```python
from build123d import *

# Parameters (mm, degrees)
SKETCH1_R                   = 250
SKETCH1_R_2                 = 25
BOSS_EXTRUDE1_DEPTH         = 6.35
TAP_DRILL_FOR_M4X0_7_TAP1_D = 3.3
TAP_DRILL_FOR_M6X1_0_TAP1_D = 5


with BuildPart() as part:
    # Sketch1 → Boss-Extrude1 (new body)
    with BuildSketch(Plane(origin=(0, 0, 0), x_dir=(1, 0, 0), z_dir=(0, 1, 0))):
        with Locations(Location((0, 0, 0), (0, 0, 270))):
            Circle(SKETCH1_R)
        with Locations(Location((0, 0, 0), (0, 0, 270))):
            Circle(SKETCH1_R_2, mode=Mode.SUBTRACT)
        with BuildLine():
            Line((-51.699063768, 192.943532686), (-21.846841855, 81.533523786))
            ThreePointArc((-21.846841855, 81.533523786), (-22.566264891, 74.464334994), (-27.799500104, 69.65764706))
            ThreePointArc((-27.799500104, 69.65764706), (-37.5, 64.951905284), (-46.42554187, 58.903896832))
            ThreePointArc((-46.42554187, 58.903896832), (-53.204873335, 56.775126162), (-59.686681932, 59.686681932))
            Line((-59.686681932, 59.686681932), (-141.244468918, 141.244468918))
            ThreePointArc((-141.244468918, 141.244468918), (-144.170273662, 148.565614941), (-140.882071162, 155.731313567))
            ThreePointArc((-140.882071162, 155.731313567), (-105, 181.865334795), (-64.426238133, 199.873109347))
            ThreePointArc((-64.426238133, 199.873109347), (-56.576459837, 199.137926932), (-51.699063768, 192.943532686))
        make_face(mode=Mode.SUBTRACT)
        with BuildLine():
            Line((141.244468918, 141.244468918), (59.686681932, 59.686681932))
            ThreePointArc((59.686681932, 59.686681932), (53.204873335, 56.775126162), (46.42554187, 58.903896832))
            ThreePointArc((46.42554187, 58.903896832), (37.5, 64.951905284), (27.799500104, 69.65764706))
            ThreePointArc((27.799500104, 69.65764706), (22.566264891, 74.464334994), (21.846841855, 81.533523786))
            Line((21.846841855, 81.533523786), (51.699063768, 192.943532686))
            ThreePointArc((51.699063768, 192.943532686), (56.576459837, 199.137926932), (64.426238133, 199.873109347))
            ThreePointArc((64.426238133, 199.873109347), (105, 181.865334795), (140.882071162, 155.731313567))
            ThreePointArc((140.882071162, 155.731313567), (144.170273662, 148.565614941), (141.244468918, 141.244468918))
        make_face(mode=Mode.SUBTRACT)
        with BuildLine():
            Line((192.943532686, -51.699063768), (81.533523786, -21.846841855))
            ThreePointArc((81.533523786, -21.846841855), (75.771138227, -17.689208833), (74.225041974, -10.753750228))
            ThreePointArc((74.225041974, -10.753750228), (75, 0), (74.225041974, 10.753750228))
            ThreePointArc((74.225041974, 10.753750228), (75.771138227, 17.689208833), (81.533523786, 21.846841855))
            Line((81.533523786, 21.846841855), (192.943532686, 51.699063768))
            ThreePointArc((192.943532686, 51.699063768), (200.746733498, 50.572311991), (205.308309294, 44.14179578))
            ThreePointArc((205.308309294, 44.14179578), (210, 0), (205.308309294, -44.14179578))
            ThreePointArc((205.308309294, -44.14179578), (200.746733498, -50.572311991), (192.943532686, -51.699063768))
        make_face(mode=Mode.SUBTRACT)
        with BuildLine():
            Line((51.699063768, -192.943532686), (21.846841855, -81.533523786))
            ThreePointArc((21.846841855, -81.533523786), (22.566264891, -74.464334994), (27.799500104, -69.65764706))
            ThreePointArc((27.799500104, -69.65764706), (37.5, -64.951905284), (46.42554187, -58.903896832))
            ThreePointArc((46.42554187, -58.903896832), (53.204873335, -56.775126162), (59.686681932, -59.686681932))
            Line((59.686681932, -59.686681932), (141.244468918, -141.244468918))
            ThreePointArc((141.244468918, -141.244468918), (144.170273662, -148.565614941), (140.882071162, -155.731313567))
            ThreePointArc((140.882071162, -155.731313567), (105, -181.865334795), (64.426238133, -199.873109347))
            ThreePointArc((64.426238133, -199.873109347), (56.576459837, -199.137926932), (51.699063768, -192.943532686))
        make_face(mode=Mode.SUBTRACT)
        with BuildLine():
            Line((-141.244468918, -141.244468918), (-59.686681932, -59.686681932))
            ThreePointArc((-59.686681932, -59.686681932), (-53.204873335, -56.775126162), (-46.42554187, -58.903896832))
            ThreePointArc((-46.42554187, -58.903896832), (-37.5, -64.951905284), (-27.799500104, -69.65764706))
            ThreePointArc((-27.799500104, -69.65764706), (-22.566264891, -74.464334994), (-21.846841855, -81.533523786))
            Line((-21.846841855, -81.533523786), (-51.699063768, -192.943532686))
            ThreePointArc((-51.699063768, -192.943532686), (-56.576459837, -199.137926932), (-64.426238133, -199.873109347))
            ThreePointArc((-64.426238133, -199.873109347), (-105, -181.865334795), (-140.882071162, -155.731313567))
            ThreePointArc((-140.882071162, -155.731313567), (-144.170273662, -148.565614941), (-141.244468918, -141.244468918))
        make_face(mode=Mode.SUBTRACT)
        with BuildLine():
            Line((-192.943532686, 51.699063768), (-81.533523786, 21.846841855))
            ThreePointArc((-81.533523786, 21.846841855), (-75.771138227, 17.689208833), (-74.225041974, 10.753750228))
            ThreePointArc((-74.225041974, 10.753750228), (-75, 0), (-74.225041974, -10.753750228))
            ThreePointArc((-74.225041974, -10.753750228), (-75.771138227, -17.689208833), (-81.533523786, -21.846841855))
            Line((-81.533523786, -21.846841855), (-192.943532686, -51.699063768))
            ThreePointArc((-192.943532686, -51.699063768), (-200.746733498, -50.572311991), (-205.308309294, -44.14179578))
            ThreePointArc((-205.308309294, -44.14179578), (-210, 0), (-205.308309294, 44.14179578))
            ThreePointArc((-205.308309294, 44.14179578), (-200.746733498, 50.572311991), (-192.943532686, 51.699063768))
        make_face(mode=Mode.SUBTRACT)
    extrude(amount=-BOSS_EXTRUDE1_DEPTH)

    # Tap Drill for M4x0.7 Tap1 (through all)
    with Locations(Plane(origin=(0, 0, -196), x_dir=(0, 0, 1), z_dir=(0, 1, 0))):
        with Locations((0, 0), (98, -169.740979142), (98, 169.740979142), (294, 169.740979142), (294, -169.740979142), (392, 0)):
            Hole(TAP_DRILL_FOR_M4X0_7_TAP1_D / 2)

    # Tap Drill for M6x1.0 Tap1 (through all)
    with Locations(Plane(origin=(0, 0, -230), x_dir=(0, 0, 1), z_dir=(0, 1, 0))):
        with Locations((0, 0), (67.365440327, 162.634559673), (230, 230), (230, -230), (67.365440327, -162.634559673), (460, 0), (392.634559673, -162.634559673), (392.634559673, 162.634559673)):
            Hole(TAP_DRILL_FOR_M6X1_0_TAP1_D / 2)


solid = part.part
```
Build history of the part. All positions in model axes, mm. A direction names the side the tool comes from. Give positions to 0.01 mm unless a question says otherwise; leave off trailing zeros. Loops run counter-clockwise (first coordinate to the right, second up) from the corner with the lowest first, then second, coordinate; pieces in that order, holes last.
Item 1: Pull direction Z, two halves, no side cores. Call faces 1 (the face through (-136.459, -3.131, 36.564)), 2 (the face through (4, -6.35, 52)), 3 (the face through (10.99, -3.13, -249.76)): released by +Z, released by -Z, zero draft, split by the parting line, or undercut.
Answers follow:
face 1: undercut
face 2: zero draft
face 3: split by the parting line
Item 2: Which spindle directions (+Z, -Z, +X, -X, +Y, -Y) get a long thin tool onto all of the face, cutting with end or side? Do faces 4 (the face through (-37.369, -3.131, -65.027)), 5 (the face through (4, 0, 52)). Say none if no direction does.
Answers follow:
face 4: +Y, -Y
face 5: +Z, -Z, +X, -X, +Y
Item 3: Slice it at B-B, the plane x = 184.5. List the corners of the cut face in (y, z).
Answers follow:
outline: (-6.35, -168.7) - (0, -168.7) - (0, -49.44) - (-6.35, -49.44) - close; (-6.35, 49.44) - (0, 49.44) - (0, 168.7) - (-6.35, 168.7) - close
Item 4: Slice it at A-A, the plane z = -174. List the corners of the cut face in (x, y), and give its area (3 significant figures).
Answers follow:
outline: (-179.51, -6.35) - (-117.58, -6.35) - (-117.58, 0) - (-179.51, 0) - close; (-46.62, -6.35) - (46.62, -6.35) - (46.62, 0) - (-46.62, 0) - close; (117.58, -6.35) - (179.51, -6.35) - (179.51, 0) - (117.58, 0) - close
area: 1,380 mm2
Item 5: Drill centre lines: line 1 (X direction, y = -2.5, z = -96); line 2 (X direction, y = -3.5, z = -15.5); line 3 (Z direction, x = -89.5, y = -5). Where is each one in solid material? Low to high.
Answers follow:
line 1: x = -230.83 to -96, -25.72 to 25.72, 96 to 230.83
line 2: x = -249.52 to -209.43, -74.69 to -19.62, 19.62 to 74.69, 209.43 to 249.52
line 3: z = -233.43 to -189.97, -89.5 to -23.98, 23.98 to 89.5, 189.97 to 233.43
Item 6: Slice it at D-D, the plane z = 127.5. List the corners of the cut face in (x, y), and give its area (3 significant figures).
Answers follow:
outline: (-215.04, -6.35) - (-127.5, -6.35) - (-127.5, 0) - (-215.04, 0) - close; (-34.16, -6.35) - (34.16, -6.35) - (34.16, 0) - (-34.16, 0) - close; (127.5, -6.35) - (215.04, -6.35) - (215.04, 0) - (127.5, 0) - close
area: 1,550 mm2
Item 7: Flat gauge pins, fed straight in: pin 1 (3 mm diameter, centred on x = 169.74, z = -98, fed in from -Y); pin 2 (1.5 mm diameter, centred on x = -160.5, y = -3, fed in from +Z); pin 3 (1 mm diameter, centred on x = 108.5, y = -3.5, fed in from -Z); pin 4 (1.5 mm diameter, centred on y = -1, z = 117.5, fed in from +X). Where does each tip first touch, or does it go through?
Answers follow:
pin 1: passes through
pin 2: stops at z = 192.3
pin 3: stops at z = -225.47
pin 4: stops at x = 221.06
Item 8: Slice it at C-C, the plane x = -180. List the corners of the cut face in (y, z), and give its area (3 significant figures).
Answers follow:
outline: (-6.35, -173.49) - (0, -173.49) - (0, -48.23) - (-6.35, -48.23) - close; (-6.35, 48.23) - (0, 48.23) - (0, 173.49) - (-6.35, 173.49) - close
area: 1,590 mm2
